Read the model definition and answer for the solid it produces. Units are mm, in the model's axes. A direction names the side the tool comes from. Coordinates: 2 decimals unless noted, no trailing zeros. Write each loop counter-clockwise with the first axis right and the second up, starting at its lowest first coordinate (ties: lowest second). Pieces come first, ordered by that corner, then holes. Notation, with made-up numbers: (-1, 66) -> (19, 66) arc R14 cw to (19, 82) -> close; hole circle Ø4 at (9, 4). An arc over 180 degrees is marked (long way). One line per item, written item: value. Start each with the question number.
1. For a pull along Z with two mould halves and no side action, classify faces 4 (the flat face through (-8, 0, -5)), 5 (the flat face through (8, 6.5, -7)), 6 (the cylindrical face through (-12.65, 3.54, -8.06)) as pulls with the +Z half, pulls with the -Z half, needs draft (parallel to the pull), parting line crosses it, or undercut.
2. For faces 1 (the cylindrical face through (-10.31, 6.75, 1.35)), 2 (the cylindrical face through (13.277, 0.246, 2.948)), 3 (the flat face through (-8, 7, 5)), determine the directions among +Z, -Z, +X, -X, +Y, -Y from which every point of the face is accessible in a straight line to the end or side of a thin tool.
3. Consider line 1 along X through (y, z) = (4.6, 0); line 2 along X through (y, z) = (0.3, 0). Determine where each line is inside the solid, lowest interval first.
4. Find section C-C, the plane y = 6. Write down the section's boundary in (x, z), and give its area (3 significant figures).
5. Given P1, Ø2, axis at x = -6, z = 11.5, coming from the -Y side; P2, Ø4, axis at x = -6, y = 4, coming from the -Z side, each flat-ended and moving along its own axis, determine where each tip first touches the part or whether it passes through.
```python
from build123d import *

# Parameters (mm, degrees)
VERRUNDUNG1_R = 0.5


with BuildPart() as part:
    # Skizze1 → Rotation1 (revolve)
    with BuildSketch(Plane.XY, mode=Mode.PRIVATE) as rotation1_sk:
        Polygon((8.5, 0), (10.4, 0), (10.4, 0.5), (13.6, 0.5), (13.6, 0), (15, 0), (15, 7), (13.6, 7), (13.6, 6.5), (10.4, 6.5), (10.4, 7), (8.5, 7), align=None)
    revolve(rotation1_sk.sketch.rotate(Axis((0, 0, 0), (0, 1, 0)), 90), axis=Axis((0, 0, 0), (0, 1, 0)))

    # Verrundung1
    verrundung1_edges = [part.edges().sort_by_distance(p)[0] for p in [
        (0, 7, 15),
        (0, 0, 15),
        (0, 0, 8.5),
        (0, 7, 8.5),
    ]]
    fillet(verrundung1_edges, radius=VERRUNDUNG1_R)


solid = part.part
```
Answer block:
1. face 4: needs draft
1. face 5: undercut
1. face 6: parting line crosses it
2. face 1: +Y
2. face 2: -Y
2. face 3: +Z, -Z, +X, -X, +Y
3. line 1: x = -15 to -8.5, 8.5 to 15
3. line 2: x = -14.96 to -13.6, -10.4 to -8.54, 8.54 to 10.4, 13.6 to 14.96
4. outline: circle Ø30 at (0, 0); hole circle Ø17 at (0, 0)
4. area: 480 mm2
5. P1: stops at y = 0
5. P2: stops at z = -14.46
